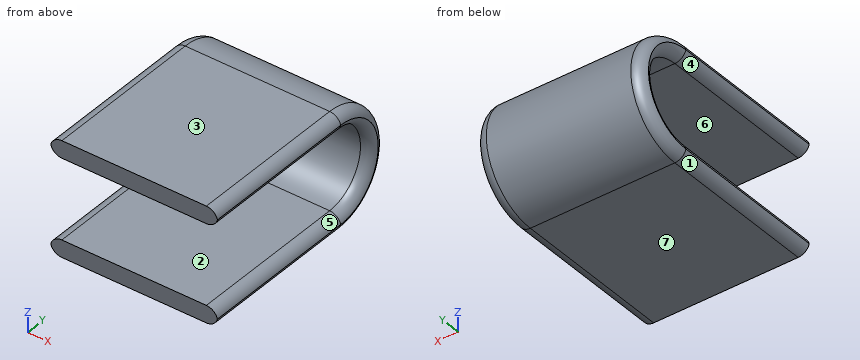
```python
from build123d import *

# Parameters (mm, degrees)
SKETCH1_W           = 18.542
SKETCH1_H           = 17.78
BOSS_EXTRUDE4_DEPTH = 1.905
SKETCH4_W           = 18.542
SKETCH4_H           = 17.78
BOSS_EXTRUDE5_DEPTH = 1.905
BOSS_EXTRUDE6_DEPTH = 18.542
FILLET1_R           = 1.27


with BuildPart() as part:
    # Sketch1 → Boss-Extrude4 (new body)
    with BuildSketch(Plane.XY):
        Rectangle(SKETCH1_W, SKETCH1_H)
    extrude(amount=-BOSS_EXTRUDE4_DEPTH)



with BuildPart() as body_2:
    # Sketch4 → Boss-Extrude5 (new body)
    with BuildSketch(Plane.XY.offset(-12.7)):
        Rectangle(SKETCH4_W, SKETCH4_H)
    extrude(amount=BOSS_EXTRUDE5_DEPTH)


with BuildPart() as part_1:
    add(part.part)

    add(body_2.part)  # Boss-Extrude6 merges body 2
    # Sketch6 → Boss-Extrude6 (add)
    with BuildSketch(Plane.ZY.offset(9.271)):
        with BuildLine():
            Line((-12.7, 8.89), (-10.795, 8.89))
            ThreePointArc((-10.795, 8.89), (-6.35, 13.335), (-1.905, 8.89))
            Line((-1.905, 8.89), (0, 8.89))
            ThreePointArc((0, 8.89), (-6.35, 15.24), (-12.7, 8.89))
        make_face()
    extrude(amount=-BOSS_EXTRUDE6_DEPTH)

    # Fillet1
    # the kernel refuses this fillet: 1.27 mm, written as the material it takes off along each edge
    with BuildSketch(Plane(origin=(9.271, 8.89, -6.35), x_dir=(0, 0, -1), z_dir=(0, -1, 0))) as fillet1_piece_1:
        with BuildLine():
            CenterArc((4.445 + FILLET1_R, -FILLET1_R), FILLET1_R, 90, 90)
            Line((4.445, -FILLET1_R), (4.445, 0))
            Line((4.445, 0), (4.445 + FILLET1_R, 0))
        make_face()
    revolve(axis=Axis((9.271, 8.89, -6.35), (1, 0, 0)), revolution_arc=180, mode=Mode.SUBTRACT)
    with BuildSketch(Plane(origin=(-9.271, 8.89, -6.35), x_dir=(0, 0, -1), z_dir=(0, -1, 0))) as fillet1_piece_2:
        with BuildLine():
            CenterArc((4.445 + FILLET1_R, FILLET1_R), FILLET1_R, 180, 90)
            Line((4.445, FILLET1_R), (4.445, 0))
            Line((4.445, 0), (4.445 + FILLET1_R, 0))
        make_face()
    revolve(axis=Axis((-9.271, 8.89, -6.35), (1, 0, 0)), revolution_arc=180, mode=Mode.SUBTRACT)
    with BuildSketch(Plane(origin=(9.271, 8.89, -6.35), x_dir=(0, 0, 1), z_dir=(0, -1, 0))) as fillet1_piece_3:
        with BuildLine():
            CenterArc((6.35 - FILLET1_R, FILLET1_R), FILLET1_R, 270, 90)
            Line((6.35, FILLET1_R), (6.35, 0))
            Line((6.35, 0), (6.35 - FILLET1_R, 0))
        make_face()
    revolve(axis=Axis((9.271, 8.89, -6.35), (-1, 0, 0)), revolution_arc=180, mode=Mode.SUBTRACT)
    with BuildSketch(Plane(origin=(-9.271, 8.89, -6.35), x_dir=(0, 0, 1), z_dir=(0, -1, 0))) as fillet1_piece_4:
        with BuildLine():
            CenterArc((6.35 - FILLET1_R, -FILLET1_R), FILLET1_R, 0, 90)
            Line((6.35, -FILLET1_R), (6.35, 0))
            Line((6.35, 0), (6.35 - FILLET1_R, 0))
        make_face()
    revolve(axis=Axis((-9.271, 8.89, -6.35), (-1, 0, 0)), revolution_arc=180, mode=Mode.SUBTRACT)
    with BuildSketch(Plane(origin=(-9.271, -12.065, -12.7), x_dir=(0, 0, 1), z_dir=(0, 1, 0)), Plane(origin=(-9.271, 8.89, 0), x_dir=(0, 0, -1), z_dir=(0, -1, 0)), Plane(origin=(9.271, -12.065, 0), x_dir=(0, 0, -1), z_dir=(0, 1, 0)), Plane(origin=(9.271, 8.89, -12.7), x_dir=(0, 0, 1), z_dir=(0, -1, 0))) as fillet1_piece_5:
        with BuildLine():
            CenterArc((FILLET1_R, FILLET1_R), FILLET1_R, 180, 90)
            Line((0, FILLET1_R), (0, 0))
            Line((0, 0), (FILLET1_R, 0))
        make_face()
    extrude(amount=20.955, mode=Mode.SUBTRACT)
    with BuildSketch(Plane(origin=(-9.271, -12.065, -10.795), x_dir=(0, 0, -1), z_dir=(0, 1, 0)), Plane(origin=(-9.271, 8.89, -1.905), x_dir=(0, 0, 1), z_dir=(0, -1, 0)), Plane(origin=(9.271, -12.065, -1.905), x_dir=(0, 0, 1), z_dir=(0, 1, 0)), Plane(origin=(9.271, 8.89, -10.795), x_dir=(0, 0, -1), z_dir=(0, -1, 0))) as fillet1_piece_6:
        with BuildLine():
            CenterArc((FILLET1_R, -FILLET1_R), FILLET1_R, 90, 90)
            Line((0, -FILLET1_R), (0, 0))
            Line((0, 0), (FILLET1_R, 0))
        make_face()
    extrude(amount=20.955, mode=Mode.SUBTRACT)


solid = part_1.part
```
Design review of the part built by this model. Coordinates are the model's own, in mm. Face numbers are marked on the shaded views. A direction names the side the tool comes from. Give positions to 0.01 mm unless a question says otherwise; leave off trailing zeros. Order: outer loops, then holes, each group sorted by start corner. A loop starts at its lowest first (then second) coordinate and runs counter-clockwise, first axis right, second up. Notation, with made-up numbers: (12, 74) -> (16, 74) arc R8 ccw to (16, 83) -> close; hole circle Ø10 at (-2.75, -26.75). An arc over 180 degrees is marked (long way). Write each question's results on one line, items separated by ' | '. Start each with the question number.
Q1. Machinability: for the marked faces 4, 5, 6 and 7, which of the approach directions +Z, -Z, +X, -X, +Y, -Y give a long, thin tool a straight path to every point of the face, cutting with its end or side? Answer none if there is none.
Q2. Add section C-C on z = -6.35. Give the boundary of the cut face in (x, y) (1 decimal).
Q3. Wall thickness on L1, parallel to Z at x = -0.5, y = 3 (3 decimals); L2, parallel to Y at x = 6, z = -6.25; L3, parallel to Z at x = -3, y = 13: over which ranges is each line inside the solid? List them lowest first. Write a range as from..to.
Q4. Add section B-B on x = -5.75. Give the boundary of the cut face in (y, z) (3 decimals), and give its area (3 significant figures).
Q5. Mouldability with a two-part tool opening along Z and no side actions: class the marked faces 1, 2 and 3 as +Z half, -Z half, draft (parallel to the pull), parting line (faces both ways), or undercut.
Q6. For pin 1 (5 mm diameter, centred on x = -1.5, z = -6, fed in from -Y); pin 2 (3 mm diameter, centred on x = 2.5, z = -7.5, fed in from -Y); pin 3 (1 mm diameter, centred on x = 6, z = -3, fed in from +Y), all flat-tipped, find the tip position at first contact; note any pin that passes through.
Q7. Add section A-A on y = -6.25. Give the boundary of the cut face in (x, z) (1 decimal), and give its area (3 significant figures).
Found:
1) face 4: -X, -Y | face 5: +X, -Y | face 6: +X, -X, -Y | face 7: -Z, +X, -X, +Y, -Y
2) outline: (-9.2, 14.3) arc R1.3 ccw to (-8, 13.3) -> (8, 13.3) arc R1.3 ccw to (9.2, 14.3) arc R1.3 ccw to (8, 15.2) -> (-8, 15.2) arc R1.3 ccw to start
3) L1: z = -12.7..-10.795, -1.905..0 | L2: y = 13.33..15.24 | L3: z = -11.19..-8.04, -4.66..-1.51
4) outline: (-8.89, -12.7) -> (8.89, -12.7) arc R6.35 ccw to (8.89, 0) -> (-8.89, 0) -> (-8.89, -1.905) -> (8.89, -1.905) arc R4.445 cw to (8.89, -10.795) -> (-8.89, -10.795) -> close | area: 100 mm2
5) face 1: -Z half | face 2: undercut | face 3: +Z half
6) pin 1: stops at y = 12.3 | pin 2: stops at y = 12.46 | pin 3: stops at y = 14.56
7) outline: (-9.2, -11.7) arc R1.3 ccw to (-8, -12.7) -> (8, -12.7) arc R1.3 ccw to (9.2, -11.7) arc R1.3 ccw to (8, -10.8) -> (-8, -10.8) arc R1.3 ccw to start; (-9.2, -1) arc R1.3 ccw to (-8, -1.9) -> (8, -1.9) arc R1.3 ccw to (9.2, -1) arc R1.3 ccw to (8, 0) -> (-8, 0) arc R1.3 ccw to start | area: 67.9 mm2
